Geometry: final body of the model. Coordinates: model frame, mm. Face numbers are marked on the shaded views. A direction names the side the tool comes from. Coordinates: 2 decimals unless noted, no trailing zeros. Loops run counter-clockwise (first coordinate to the right, second up) from the corner with the lowest first, then second, coordinate; pieces in that order, holes last. Notation, with made-up numbers: (8.25, 52.25) - (35.25, 52.25) arc R29 ccw to (35.25, 83.25) - close; hole circle Ø7 at (15.25, 42). An arc over 180 degrees is marked (long way). Put each result on its own line as item: value. Start each with the question number.
1) Draft query along Z for the marked faces 3, 4 and 5. Return one class per face: +Z half, -Z half, draft (parallel to the pull), parting line (faces both ways), or undercut.
2) Reachability of the marked faces 1 and 2 from +Z, -Z, +X, -X, +Y, -Y: full face, straight path, thin tool, end or side. Return the list, or none.
3) Section A-A on z = -8. Output: boundary loops of the cut face in (x, y) (3 decimals), and give its area (3 significant figures).
4) Section D-D on z = -88. Output: boundary loops of the cut face in (x, y), and give its area (3 significant figures).
5) Contact query for flat-ended pins moving along their axis: pin 1 Ø7 at (y, z) = (0, -8) entering from +X; pin 2 Ø6 at (y, z) = (2, -9.5) entering from -X; pin 3 Ø10 at (x, z) = (1.5, -32.5) entering from -Y. Output: stop coordinate, or through.
6) Material intervals for line 1 along Z through (x, y) = (-2.25, 0); line 2 along Z through (x, y) = (-4.5, 2.75); line 3 along Z through (x, y) = (3.25, -5.25), sorted ascending. Write a range as from..to.
7) Section B-B on y = 0. Output: boundary loops of the cut face in (x, z).
8) Section C-C on x = 0. Output: boundary loops of the cut face in (y, z).
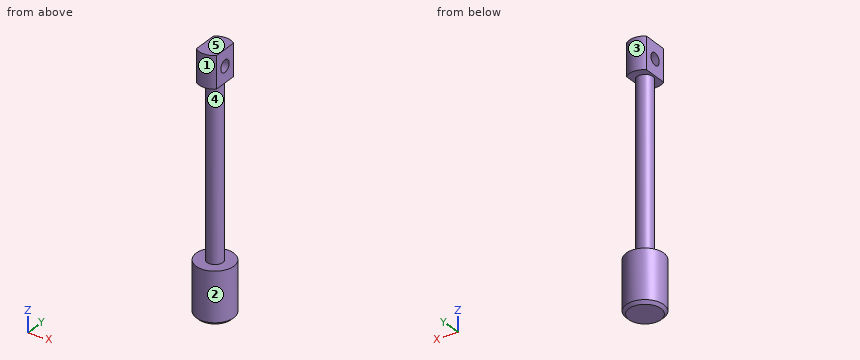
```python
from build123d import *

# Parameters (mm, degrees)
ENL_V_START             = -16
ENL_V_MAT_EXTRU_1_DEPTH = 16
ENL_V_MAT_EXTRU_2_REACH = 131.153
ESQUISSE3_R             = 3


with BuildPart() as part:
    # Esquisse1 → Révolution1 (revolve)
    with BuildSketch(Plane(origin=(0, 0, 0), x_dir=(1, 0, 0), z_dir=(0, 1, 0))):
        Polygon((0, 0), (-8, 0), (-8, 16), (-4, 16), (-4, 102), (-9.414213562, 102), (-9.414213562, 126.585786438), (-8, 128), (0, 128), align=None)
    revolve(axis=Axis((0, 0, -128), (0, 0, 1)))

    # Esquisse2 → Enlèv. mat.-Extru.1 (cut)
    with BuildSketch(Plane.XY.offset(ENL_V_START)):
        Polygon((-5, 10), (-5, -12), (5, -12), (5, 10), (12, 10), (12, -15), (-12, -15), (-12, 10), align=None)
    extrude(amount=ENL_V_MAT_EXTRU_1_DEPTH, mode=Mode.SUBTRACT)

    # Esquisse3 → Enlèv. mat.-Extru.2 (cut, up to next)
    with BuildSketch(Plane.ZY.offset(5), mode=Mode.PRIVATE) as enl_v_mat_extru_2_sk1:
        with Locations(Location((-8, 0, 0), (0, 0, 270))):
            Circle(ESQUISSE3_R)
    enl_v_mat_extru_2_tool1 = extrude(enl_v_mat_extru_2_sk1.sketch, amount=-ENL_V_MAT_EXTRU_2_REACH, mode=Mode.PRIVATE) & part.part
    add(enl_v_mat_extru_2_tool1.solids().sort_by_distance((-5, 0, -8))[0], mode=Mode.SUBTRACT)


solid = part.part
```
Answer block:
1. face 3: draft
1. face 4: undercut
1. face 5: +Z half
2. face 1: +Z, -Y
2. face 2: +Z, -Z
3. outline: (-5, -6.245) arc R8 ccw to (5, -6.245) - (5, -3) - (-5, -3) - close; (-5, 3) - (5, 3) - (5, 6.245) arc R8 ccw to (-5, 6.245) - close
3. area: 88.9 mm²
4. outline: circle Ø8 at (0, 0)
4. area: 50.3 mm²
5. pin 1: stops at x = 5
5. pin 2: stops at x = -5
5. pin 3: stops at y = -4
6. line 1: z = -128..-11, -5..0
6. line 2: z = -128..-102, -16..-9.2, -6.8..0
6. line 3: z = -128..-102, -16..0
7. outline: (-9.41, -126.59) - (-8, -128) - (8, -128) - (9.41, -126.59) - (9.41, -102) - (4, -102) - (4, -16) - (5, -16) - (5, -11) - (-5, -11) - (-5, -16) - (-4, -16) - (-4, -102) - (-9.41, -102) - close; (-5, -5) - (5, -5) - (5, 0) - (-5, 0) - close
8. outline: (-9.41, -126.59) - (-8, -128) - (8, -128) - (9.41, -126.59) - (9.41, -102) - (4, -102) - (4, -16) - (8, -16) - (8, 0) - (-8, 0) - (-8, -16) - (-4, -16) - (-4, -102) - (-9.41, -102) - close; hole circle Ø6 at (0, -8)
